The listing builds one solid part. Answer for the finished solid, in the listing's coordinates (mm). Give positions to 0.01 mm unless a question says otherwise; leave off trailing zeros. Write each loop counter-clockwise with the first axis right and the second up, starting at its lowest first coordinate (ties: lowest second). Pieces come first, ordered by that corner, then holes. Notation, with made-up numbers: M 24,86 L 79,86 A19 ccw 79,94 Z; hole C 84.25,38 d4. An arc over 180 degrees is marked long. Answer as a JSON object with one key per item and string values.
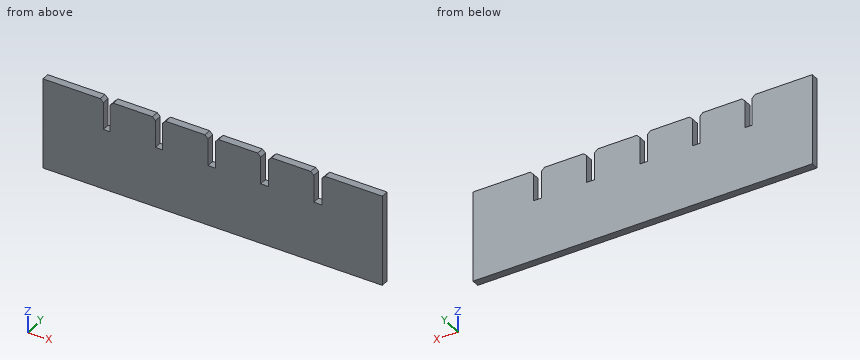
Autodesk Inventor part; units mm, degrees
ref_plane "YZ Plane" through (0, 0, 0) normal (1, 0, 0) x (0, 1, 0)
ref_plane "XZ Plane" through (0, 0, 0) normal (0, 1, 0) x (-1, 0, 0)
ref_plane "XY Plane" through (0, 0, 0) normal (0, 0, 1) x (1, 0, 0)
sketch "Sketch1" plane through (0, 0, 0) normal (0, 1, 0) x (-1, 0, 0)
  line L0 (75, -15) -> (-75, -15)
  line L1 (-75, -15) -> (-75, 15)
  line L2 (-75, 15) -> (75, 15)
  line L3 (75, 15) -> (75, -15)
  point P0 (0, 0)
  point P1 (0, -15)
  point P2 (75, 0)
  point P3 (0, 15)
  dimension "d0" = 150
  dimension "d1" = 30
extrude "Extrusion1" add sketch "Sketch1" along normal blind 2.5
sketch "Sketch3" plane through (0, 2.5, 0) normal (0, 1, 0) x (1, 0, 0)
  line L0 (-75, 15) -> (-75, -15)
  line L1 (-75, -15) -> (75, -15)
  line L2 (-55, -15) -> (-52.7, -15)
  line L3 (-52.7, -15) -> (-52.7, -5)
  line L4 (-52.7, -5) -> (-55, -5)
  line L5 (-55, -5) -> (-55, -15)
  point P0 (0, 0)
  point P1 (-53.85, -15)
  point P2 (0, -15)
  dimension "d4" = 2.3
  dimension "d5" = 10
  dimension "d6" = 20
extrude "-0.2" cut sketch "Sketch3" along normal through all both and the other way through all
sketch "Sketch4" plane through (0, 2.5, 0) normal (0, 1, 0) x (1, 0, 0)
  line L0 (-75, -15) -> (-55, -15)
  line L1 (-37.7, -5) -> (-35.3, -5)
  line L2 (-35.3, -5) -> (-35.3, -15)
  line L3 (-35.3, -15) -> (-37.7, -15)
  line L4 (-37.7, -15) -> (-37.7, -5)
  point P0 (-52.7, -15)
  point P1 (0, 0)
  point P2 (-36.5, -15)
  point P3 (-65, -15)
  dimension "d9" = 10
  dimension "d10" = 2.4
  dimension "d11" = 15
extrude "-0.1" cut sketch "Sketch4" against normal through all
sketch "Sketch5" plane through (0, 2.5, 0) normal (0, 1, 0) x (1, 0, 0)
  line L0 (-75, -15) -> (-55, -15)
  line L1 (-20.3, -5) -> (-17.8, -5)
  line L2 (-17.8, -5) -> (-17.8, -15)
  line L3 (-17.8, -15) -> (-20.3, -15)
  line L4 (-20.3, -15) -> (-20.3, -5)
  point P0 (-35.3, -5)
  point P1 (0, 0)
  point P2 (-19.05, -15)
  point P3 (-65, -15)
  dimension "d15" = 10
  dimension "d16" = 2.5
  dimension "d17" = 15
extrude "0.0" cut sketch "Sketch5" against normal through all
sketch "Sketch6" plane through (0, 2.5, 0) normal (0, 1, 0) x (1, 0, 0)
  line L0 (-75, -15) -> (-55, -15)
  line L1 (-2.8, -15) -> (-0.2, -15)
  line L2 (-0.2, -15) -> (-0.2, -5)
  line L3 (-0.2, -5) -> (-2.8, -5)
  line L4 (-2.8, -5) -> (-2.8, -15)
  point P0 (-17.8, -5)
  point P1 (0, 0)
  point P2 (-1.5, -15)
  point P3 (-65, -15)
  dimension "d20" = 10
  dimension "d21" = 2.6
  dimension "d22" = 15
extrude "+0.1" cut sketch "Sketch6" against normal through all
sketch "Sketch7" plane through (0, 2.5, 0) normal (0, 1, 0) x (1, 0, 0)
  line L0 (-75, -15) -> (-55, -15)
  line L1 (14.8, -15) -> (17.5, -15)
  line L2 (17.5, -15) -> (17.5, -5)
  line L3 (17.5, -5) -> (14.8, -5)
  line L4 (14.8, -5) -> (14.8, -15)
  point P0 (-0.2, -5)
  point P1 (0, 0)
  point P2 (16.15, -15)
  point P3 (-65, -15)
  dimension "d25" = 10
  dimension "d26" = 2.7
  dimension "d27" = 15
extrude "+0.2" cut sketch "Sketch7" against normal through all
sketch "Sketch8" plane through (0, 2.5, 0) normal (0, 1, 0) x (1, 0, 0)
  line L0 (75, 15) -> (-75, 15)
  line L1 (-75, 15) -> (-75, -15)
  line L2 (-75, -15) -> (-55, -15)
  line L3 (-75, 15) -> (37.5, 15)
  line L4 (37.5, 15) -> (37.5, -15)
  line L5 (37.5, -15) -> (-75, -15)
  line L6 (-75, -15) -> (-75, 15)
  point P0 (17.5, -5)
  point P1 (0, 0)
  point P2 (-18.75, -15)
  point P3 (-65, -15)
  point P4 (-18.75, 15)
  point P5 (0, 15)
  point P6 (-75, 0)
  point P7 (-75, 0)
  dimension "d30" = 20
extrude "Extrusion7" cut sketch "Sketch8" against normal through all keep common part
chamfer "Chamfer1" distance 1 angle 45 10 edges at (-55, 1.25, 15) (-52.7, 1.25, 15) (-37.7, 1.25, 15) (-35.3, 1.25, 15) (-20.3, 1.25, 15) (-17.8, 1.25, 15) (-2.8, 1.25, 15) (-0.2, 1.25, 15) (14.8, 1.25, 15) (17.5, 1.25, 15)
equation "\"d2\" = CardThickness"
equation "\"d12\" = CardThickness"
equation "\"d16\" = CardThickness"
equation "\"d18\" = CardThickness"
equation "\"d23\" = CardThickness"
equation "\"d28\" = CardThickness"
equation "\"d31\" = CardThickness"
equation "\"CardThickness\" = 2.5"
properties part number "SlotRuler"
1. A flat-ended cylindrical pin translates along its axis: pin 1 (1.2 mm diameter, centred on x = 15.5, y = 1.5, fed in from +Z). Find the tip coordinate at first contact, or state that the pin passes through.
Verdict:
{"pin 1": "stops at z = 5"}
2. A cutting plane is placed at A-A, the plane z = 12.5. Give the vertices of the cut face in (x, y), plus the area to 3 significant figures.
Verdict:
{"outline": "M -75,0 L -55,0 L -55,2.5 L -75,2.5 Z; M -52.7,0 L -37.7,0 L -37.7,2.5 L -52.7,2.5 Z; M -35.3,0 L -20.3,0 L -20.3,2.5 L -35.3,2.5 Z; M -17.8,0 L -2.8,0 L -2.8,2.5 L -17.8,2.5 Z; M -0.2,0 L 14.8,0 L 14.8,2.5 L -0.2,2.5 Z; M 17.5,0 L 37.5,0 L 37.5,2.5 L 17.5,2.5 Z", "area": "250 mm2"}
3. Consider line 1 along X through (y, z) = (0.2, 12); line 2 along Z through (x, y) = (16, 1.1); line 3 along Z through (x, y) = (0.5, 0.8). Determine where each line is inside the solid, lowest interval first.
Verdict:
{"line 1": "x = -75 to -55, -52.7 to -37.7, -35.3 to -20.3, -17.8 to -2.8, -0.2 to 14.8, 17.5 to 37.5", "line 2": "z = -15 to 5", "line 3": "z = -15 to 14.7"}
